from build123d import *

# Parameters (mm, degrees)
F1_DEPTH = 54
F2_DEPTH = 10
F3_START = 10
F3_DEPTH = 44
F5_DEPTH = 95.001
F6_W     = 10
F6_H     = 50
F6_W_2   = 12
F7_DEPTH = 114
F8_R     = 11.1
F9_DEPTH = 22.001


with BuildPart() as f1:
    # F0 (on Front) → F1 (new body)
    with BuildSketch(Plane.XZ):
        with BuildLine():
            ThreePointArc((-23.6755279772, 16), (0, 28.575), (23.6755279772, 16))
            Line((23.6755279772, 16), (51.5751878329, 16))
            ThreePointArc((51.5751878329, 16), (45.1247409006, 29.6607106903), (35.1425667816, 41))
            ThreePointArc((35.1425667816, 41), (-14.9585346426, 51.8868214612), (-51.5751878329, 16))
            Line((-51.5751878329, 16), (-23.6755279772, 16))
        make_face()
        with BuildLine():
            Line((51.5751878329, -16), (23.6755279772, -16))
            ThreePointArc((23.6755279772, -16), (0, -28.575), (-23.6755279772, -16))
            Line((-23.6755279772, -16), (-51.5751878329, -16))
            ThreePointArc((-51.5751878329, -16), (-14.9585346426, -51.8868214612), (35.1425667816, -41))
            ThreePointArc((35.1425667816, -41), (45.1247409006, -29.6607106903), (51.5751878329, -16))
        make_face()
        with BuildLine():
            ThreePointArc((23.6755279772, 16), (27.3226905424, 8.3666723687), (28.575, 0))
            ThreePointArc((28.575, 0), (27.3226905424, -8.3666723687), (23.6755279772, -16))
            Line((23.6755279772, -16), (51.5751878329, -16))
            ThreePointArc((51.5751878329, -16), (53.3903556037, -8.0913489921), (54, 0))
            ThreePointArc((54, 0), (53.3903556037, 8.0913489921), (51.5751878329, 16))
            Line((51.5751878329, 16), (23.6755279772, 16))
        make_face()
        with BuildLine():
            ThreePointArc((-23.6755279772, -16), (-28.575, 0), (-23.6755279772, 16))
            Line((-23.6755279772, 16), (-51.5751878329, 16))
            ThreePointArc((-51.5751878329, 16), (-54, 0), (-51.5751878329, -16))
            Line((-51.5751878329, -16), (-23.6755279772, -16))
        make_face()
    extrude(amount=F1_DEPTH)

    # F0 (on Front) → F2 (join)
    with BuildSketch(Plane.XZ):
        with BuildLine():
            ThreePointArc((-23.6755279772, -16), (-28.575, 0), (-23.6755279772, 16))
            Line((-23.6755279772, 16), (-51.5751878329, 16))
            ThreePointArc((-51.5751878329, 16), (-54, 0), (-51.5751878329, -16))
            Line((-51.5751878329, -16), (-23.6755279772, -16))
        make_face()
        with BuildLine():
            ThreePointArc((23.6755279772, 16), (27.3226905424, 8.3666723687), (28.575, 0))
            ThreePointArc((28.575, 0), (27.3226905424, -8.3666723687), (23.6755279772, -16))
            Line((23.6755279772, -16), (51.5751878329, -16))
            ThreePointArc((51.5751878329, -16), (53.3903556037, -8.0913489921), (54, 0))
            ThreePointArc((54, 0), (53.3903556037, 8.0913489921), (51.5751878329, 16))
            Line((51.5751878329, 16), (23.6755279772, 16))
        make_face()
    extrude(amount=-F2_DEPTH)

    # F0 (on Front) → F3 (join)
    with BuildSketch(Plane.XZ.offset(F3_START)):
        with BuildLine():
            ThreePointArc((35.1425667816, 41), (45.1247409006, 29.6607106903), (51.5751878329, 16))
            ThreePointArc((51.5751878329, 16), (53.3903556037, 8.0913489921), (54, 0))
            ThreePointArc((54, 0), (53.3903556037, -8.0913489921), (51.5751878329, -16))
            ThreePointArc((51.5751878329, -16), (45.1247409006, -29.6607106903), (35.1425667816, -41))
            Line((35.1425667816, -41), (174, -41))
            Line((174, -41), (174, 41))
            Line((174, 41), (35.1425667816, 41))
        make_face()
    extrude(amount=F3_DEPTH)

    # F4 (on face) → F5 (cut, through all)
    with BuildSketch(Plane(origin=(0, 0, -41), x_dir=(1, 0, 0), z_dir=(0, 0, -1))):
        Polygon((174, 22), (162, 10), (174, 10), align=None)
    extrude(amount=-F5_DEPTH, mode=Mode.SUBTRACT)

    # F6 (on face) → F7 (cut)
    with BuildSketch(Plane.YZ.offset(174)):
        with Locations((-27, 0)):
            Rectangle(F6_W, F6_H)
        with Locations((-16, 0)):
            Rectangle(F6_W_2, F6_H)
    extrude(amount=-F7_DEPTH, mode=Mode.SUBTRACT)

    # F8 (on face) → F9 (cut, through all)
    with BuildSketch(Plane(origin=(0, -32, 0), x_dir=(-1, 0, 0), z_dir=(0, 1, 0))):
        with Locations((-139, 0)):
            Circle(F8_R)
        with Locations((-89, 0)):
            Circle(F8_R)
    extrude(amount=-F9_DEPTH, mode=Mode.SUBTRACT)


solid = f1.part
For this review, take the finished solid that the model builds, in its own axes (mm). A direction names the side the tool comes from. Coordinates: 2 decimals unless noted, no trailing zeros. Loops run counter-clockwise (first coordinate to the right, second up) from the corner with the lowest first, then second, coordinate; pieces in that order, holes last. Notation, with made-up numbers: (-14, 34.25) - (-10, 34.25) arc R11 cw to (-10, 47.25) - close; hole circle Ø10 at (-4, -22). An arc over 180 degrees is marked (long way). Use a Markdown table: item, result. Add a question column.
Item 1: We need section C-C (z = -3.5). Give the boundary of the cut face in (x, y).
Item 2: We need section B-B (x = 139). Give the boundary of the cut face in (y, z), and give its area (3 significant figures).
Item 3: We need section D-D (y = 4). Give the boundary of the cut face in (x, z) (3 decimals), and give its area (3 significant figures).
Item 4: We need section A-A (y = -41.5). Give the boundary of the cut face in (x, z) (3 decimals).
Item 5: Tool access review of faces 5 (the face through (106, -32, 41)), 6 (the face through (104, -32, -41)), 7 (the face through (118, -32, 0)), 8 (the face through (-1, 0, -35)), 9 (the face through (-37, 5, 16)): name each direction out of +Z, -Z, +X, -X, +Y, -Y from which nothing blocks a thin tool from reaching the whole face with its end or side.
Item 6: For line 1 (Z direction, x = 139, y = -46.5); line 2 (Y direction, x = 56, z = -15.5); line 3 (X direction, y = -14.5, z = -10), list the stretches that pass through material, from the lowest coordinate up.
Item 7: Insertion check: pin 1 Ø11.5 at (x, z) = (-20.5, 31) entering from +Y; pin 2 Ø6 at (x, y) = (91.5, -25) entering from +Z; pin 3 Ø4 at (x, z) = (95.5, 3) entering from +Y; pin 4 Ø10 at (y, z) = (-14, -2.5) entering from +X. Each pin has a flat end and moves straight along its axis. Give the tip position at first contact, or say it passes through.
Item 8: Mouldability with a two-part tool opening along Z and no side actions: class faces 1 (the face through (60, -21, 0)), 2 (the face through (38, 5, 16)), 3 (the face through (58, -54, 1)), 4 (the face through (37, 5, -16)) as pulls with the +Z half, pulls with the -Z half, needs draft (parallel to the pull), parting line crosses it, or undercut.
Results list:
| question | item | result |
|---|---|---|
| 1 | outline | (-53.89, -54) - (-28.36, -54) - (-28.36, 10) - (-53.89, 10) - close; (28.36, -54) - (78.47, -54) - (78.47, -32) - (60, -32) - (60, -10) - (53.89, -10) - (53.89, 10) - (28.36, 10) - close; (99.53, -54) - (128.47, -54) - (128.47, -32) - (99.53, -32) - close; (149.53, -54) - (174, -54) - (174, -32) - (149.53, -32) - close |
| 2 | outline | (-54, -41) - (-10, -41) - (-10, -25) - (-32, -25) - (-32, -11.1) - (-54, -11.1) - close; (-54, 11.1) - (-32, 11.1) - (-32, 25) - (-10, 25) - (-10, 41) - (-54, 41) - close |
| 2 | area | 2,020 mm^2 |
| 3 | outline | (-51.575, -16) - (-23.676, -16) arc R28.575 cw to (-23.676, 16) - (-51.575, 16) arc R54 ccw to start; (23.676, -16) - (51.575, -16) arc R54 ccw to (51.575, 16) - (23.676, 16) arc R28.575 cw to start |
| 3 | area | 1,680 mm^2 |
| 4 | outline | (35.143, -41) - (174, -41) - (174, 41) - (35.143, 41) arc R54 ccw (long way) to start; hole circle Ø57.15 at (0, 0); hole circle Ø22.2 at (89, 0); hole circle Ø22.2 at (139, 0) |
| 5 | face 5 | +Z, +X, +Y, -Y |
| 5 | face 6 | -Z, +X, +Y, -Y |
| 5 | face 7 | +X, +Y |
| 5 | face 8 | -Z, +X, -X, +Y |
| 5 | face 9 | +Z, +X, -X, +Y |
| 6 | line 1 | z = -41 to -11.1, 11.1 to 41 |
| 6 | line 2 | y = -54 to -10 |
| 6 | line 3 | x = -53.07 to -26.77, 26.77 to 60 |
| 7 | pin 1 | stops at y = 0 |
| 7 | pin 2 | stops at z = 41 |
| 7 | pin 3 | passes through |
| 7 | pin 4 | stops at x = 60 |
| 8 | face 1 | undercut |
| 8 | face 2 | pulls with the +Z half |
| 8 | face 3 | needs draft |
| 8 | face 4 | pulls with the -Z half |
